from build123d import *

# Parameters (mm, degrees)
BOSS_EXTRU_1_DEPTH      = 60
ESQUISSE2_W             = 40
ESQUISSE2_H             = 86
ENL_V_MAT_EXTRU_1_DEPTH = 15
ESQUISSE3_W             = 40
ESQUISSE3_H             = 86
ENL_V_MAT_EXTRU_2_DEPTH = 15
ESQUISSE4_R             = 10
ENL_V_MAT_EXTRU_3_DEPTH = 98.462813421
ESQUISSE5_R             = 5
ENL_V_MAT_EXTRU_4_DEPTH = 129.922457314


with BuildPart() as part:
    # Esquisse1 → Boss.-Extru.1 (new body)
    with BuildSketch(Plane.XY):
        Polygon((-75, 43), (75, 43), (75, 35), (44, 4), (36, 4), (36, -4), (44, -4), (75, -35), (75, -43), (-75, -43), (-75, -35), (-44, -4), (-36, -4), (-36, 4), (-44, 4), (-75, 35), align=None)
    extrude(amount=BOSS_EXTRU_1_DEPTH)

    # Esquisse2 → Enlèv. mat.-Extru.1 (cut)
    with BuildSketch(Plane.XY.offset(60)):
        Rectangle(ESQUISSE2_W, ESQUISSE2_H)
    extrude(amount=-ENL_V_MAT_EXTRU_1_DEPTH, mode=Mode.SUBTRACT)

    # Esquisse3 → Enlèv. mat.-Extru.2 (cut)
    with BuildSketch(Plane(origin=(0, 0, 0), x_dir=(-1, 0, 0), z_dir=(0, 0, -1))):
        Rectangle(ESQUISSE3_W, ESQUISSE3_H)
    extrude(amount=-ENL_V_MAT_EXTRU_2_DEPTH, mode=Mode.SUBTRACT)

    # Esquisse4 → Enlèv. mat.-Extru.3 (cut, through all)
    with BuildSketch(Plane(origin=(0, 0, 15), x_dir=(-1, 0, 0), z_dir=(0, 0, -1))):
        Circle(ESQUISSE4_R)
    extrude(amount=-ENL_V_MAT_EXTRU_3_DEPTH, mode=Mode.SUBTRACT)

    # Esquisse5 → Enlèv. mat.-Extru.4 (cut, through all)
    with BuildSketch(Plane(origin=(0, 43, 0), x_dir=(1, 0, 0), z_dir=(0, 1, 0))):
        with Locations(Location((0, -30, 0), (0, 0, 270))):
            Circle(ESQUISSE5_R)
    extrude(amount=-ENL_V_MAT_EXTRU_4_DEPTH, mode=Mode.SUBTRACT)


solid = part.part
Geometry: final body of the model. Coordinates: model frame, mm. A direction names the side the tool comes from. Round coordinates to 2 decimals unless told otherwise and drop trailing zeros. Loops run counter-clockwise (first coordinate to the right, second up) from the corner with the lowest first, then second, coordinate; pieces in that order, holes last. Notation, with made-up numbers: M 15.5,41.25 L 30.5,41.25 A19 ccw 30.5,73.25 Z; hole C -31.5,-6 d10. An arc over 180 degrees is marked long. Put each result on its own line as item: value. Start each with the question number.
(1) Draft query along Y for faces 1 (the face through (1, -43, 36)), 2 (the face through (-59, 19, 30)), 3 (the face through (-36, 0, 30)), 4 (the face through (-20, -1, 53)). Return one class per face: +Y half, -Y half, draft (parallel to the pull), parting line (faces both ways), or undercut.
(2) Section query D-D (y = -33). Return loops of the section in (x, z).
(3) Contact query for flat-ended pins moving along their axis: pin 1 Ø6.5 at (y, z) = (1.5, 23) entering from +X; pin 2 Ø23 at (x, y) = (0, 0) entering from +Z; pin 3 Ø7.5 at (y, z) = (-17, 50.5) entering from +X; pin 4 Ø9 at (x, z) = (0, 30) entering from +Y (3 decimals). Output: stop coordinate, or through.
(4) Set-up query: faces 5 (the face through (40, -4, 30)), 6 (the face through (0.3, 10.2, 15)), 7 (the face through (-40, 4, 30)). Return all of +Z, -Z, +X, -X, +Y, -Y with unobstructed straight access to the full face (end or side cutting, diameter ignored); none if empty.
(5) Section query C-C (z = 30). Return loops of the section in (x, y), then the cut area to 3 significant figures.
(6) Section query B-B (x = 0). Return loops of the section in (y, z), then the cut area to 3 significant figures.
(7) Material intervals for line 1 along Y through (x, z) = (-40, 36.5); line 2 along Z through (x, y) = (0, -16); line 3 along Y through (x, z) = (0, 23), sorted ascending. Write a range as [from, to].
(8) Section query A-A (y = 0). Return loops of the section in (x, z).
Findings below:
1. face 1: -Y half
1. face 2: undercut
1. face 3: undercut
1. face 4: draft
2. outline: M -73,0 L -20,0 L -20,15 L 20,15 L 20,0 L 73,0 L 73,60 L 20,60 L 20,45 L -20,45 L -20,60 L -73,60 Z; hole C 0,30 d10
3. pin 1: stops at x = 44.75
3. pin 2: stops at z = 45
3. pin 3: stops at x = 60.75
3. pin 4: passes through
4. face 5: +Z, -Z, +X
4. face 6: -Z, +Y, -Y
4. face 7: +Z, -Z, -X
5. outline: M -75,-43 L -5,-43 L -5,-8.66 A10 cw -5,8.66 L -5,43 L -75,43 L -75,35 L -44,4 L -36,4 L -36,-4 L -44,-4 L -75,-35 Z; M 5,-43 L 75,-43 L 75,-35 L 44,-4 L 36,-4 L 36,4 L 44,4 L 75,35 L 75,43 L 5,43 L 5,8.66 A10 cw 5,-8.66 Z
5. area: 9,370 mm2
6. outline: M -43,15 L -10,15 L -10,25 L -43,25 Z; M -43,35 L -10,35 L -10,45 L -43,45 Z; M 10,15 L 43,15 L 43,25 L 10,25 Z; M 10,35 L 43,35 L 43,45 L 10,45 Z
6. area: 1,320 mm2
7. line 1: y = [-43, -4], [4, 43]
7. line 2: z = [15, 25], [35, 45]
7. line 3: y = [-43, -10], [10, 43]
8. outline: M -36,0 L -20,0 L -20,15 L -10,15 L -10,45 L -20,45 L -20,60 L -36,60 Z; M 10,15 L 20,15 L 20,0 L 36,0 L 36,60 L 20,60 L 20,45 L 10,45 Z
